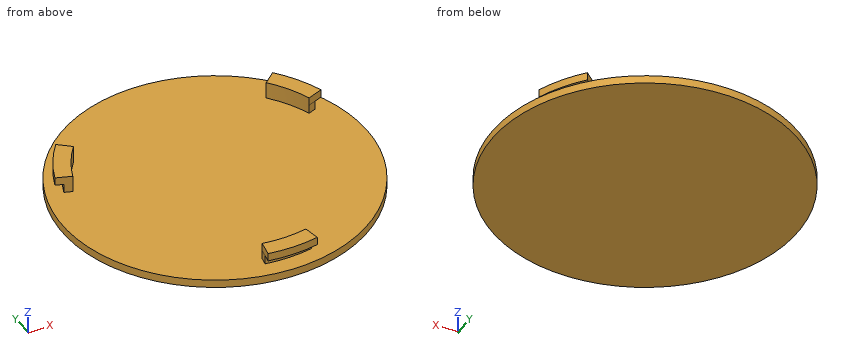
from build123d import *

# Parameters (mm, degrees)
F0_R     = 19
F1_DEPTH = 1
F3_DEPTH = 1.1
F5_DEPTH = 1


with BuildPart() as f1:
    # F0 (on Top) → F1 (new body)
    with BuildSketch(Plane.XY):
        Circle(F0_R)
    extrude(amount=F1_DEPTH)

    # F2 (on face) → F3 (join)
    with BuildSketch(Plane.XY.offset(1)):
        with BuildLine():
            Line((14.815816, 5.770752), (15.747629, 6.133693))
            ThreePointArc((15.747629, 6.133693), (14.443282, 8.775055), (12.700084, 11.149792))
            Line((12.700084, 11.149792), (11.9486, 10.490041))
            ThreePointArc((11.9486, 10.490041), (13.58865, 8.255821), (14.815816, 5.770752))
        make_face()
        with BuildLine():
            ThreePointArc((-15.058942, 5.102771), (-13.944076, 7.640206), (-12.405526, 9.945497))
            Line((-12.405526, 9.945497), (-13.185748, 10.571))
            ThreePointArc((-13.185748, 10.571), (-14.821062, 8.120722), (-16.006045, 5.4237))
            Line((-16.006045, 5.4237), (-15.058942, 5.102771))
        make_face()
        with BuildLine():
            ThreePointArc((3.110342, -15.592812), (0.355426, -15.896027), (-2.41029, -15.71625))
            Line((-2.41029, -15.71625), (-2.561881, -16.704693))
            ThreePointArc((-2.561881, -16.704693), (0.377779, -16.895777), (3.305961, -16.573492))
            Line((3.305961, -16.573492), (3.110342, -15.592812))
        make_face()
    extrude(amount=F3_DEPTH)

    # F4 (on face) → F5 (join)
    with BuildSketch(Plane.XY.offset(2.1)):
        with BuildLine():
            ThreePointArc((-15.058942, 5.102771), (-13.944076, 7.640206), (-12.405526, 9.945497))
            Line((-12.405526, 9.945497), (-13.96597, 11.196503))
            ThreePointArc((-13.96597, 11.196503), (-15.698048, 8.601238), (-16.953148, 5.744629))
            Line((-16.953148, 5.744629), (-15.058942, 5.102771))
        make_face()
        with BuildLine():
            Line((-2.41029, -15.71625), (-2.713471, -17.693136))
            ThreePointArc((-2.713471, -17.693136), (0.400133, -17.895527), (3.50158, -17.554172))
            Line((3.50158, -17.554172), (3.110342, -15.592812))
            ThreePointArc((3.110342, -15.592812), (0.355426, -15.896027), (-2.41029, -15.71625))
        make_face()
        with BuildLine():
            Line((14.815816, 5.770752), (16.679441, 6.496633))
            ThreePointArc((16.679441, 6.496633), (15.297915, 9.294289), (13.451568, 11.809543))
            Line((13.451568, 11.809543), (11.9486, 10.490041))
            ThreePointArc((11.9486, 10.490041), (13.58865, 8.255821), (14.815816, 5.770752))
        make_face()
    extrude(amount=F5_DEPTH)


solid = f1.part
Model file for the job. Use its own axes, mm. Round coordinates to 2 decimals unless told otherwise and drop trailing zeros. Loops run counter-clockwise (first coordinate to the right, second up) from the corner with the lowest first, then second, coordinate; pieces in that order, holes last. Notation, with made-up numbers: (36.5, 81.25) - (83.5, 81.25) arc R21 ccw to (83.5, 116.25) - close; hole circle Ø1 at (87, -11.75). An arc over 180 degrees is marked (long way). Write each question's results on one line, items separated by ' | '.
(1) Saw through at B-B, the plane y = 0. List the corners of the cut face in (x, z), then the cut area to 3 significant figures.
Answer below:
outline: (-19, 0) - (19, 0) - (19, 1) - (-19, 1) - close | area: 38.0 mm^2
(2) Pin check, flat tips, straight feed: pin 1 (11.5 mm diameter, centred on x = 3.5, y = 8, fed in from +Z); pin 2 (1.5 mm diameter, centred on y = 4, z = 0.5, fed in from -X). Stop position of each tip, or through.
Answer below:
pin 1: stops at z = 1 | pin 2: stops at x = -18.72
(3) Saw through at A-A, the plane x = 0. List the corners of the cut face in (y, z).
Answer below:
outline: (-19, 0) - (19, 0) - (19, 1) - (-15.9, 1) - (-15.9, 3.1) - (-17.9, 3.1) - (-17.9, 2.1) - (-16.9, 2.1) - (-16.9, 1) - (-19, 1) - close
(4) Wall check: L1, parallel to Z at x = -9, y = 1.5; L2, parallel to X at y = 12.5, z = 0.7; L3, parallel to Y at x = -1, z = 1.1. Give the ranges that are in metal, low to high.
Answer below:
L1: z = 0 to 1 | L2: x = -14.31 to 14.31 | L3: y = -16.87 to -15.87
(5) Saw through at C-C, the plane x = -7.5. List the corners of the cut face in (y, z), then the cut area to 3 significant figures.
Answer below:
outline: (-17.46, 0) - (17.46, 0) - (17.46, 1) - (-17.46, 1) - close | area: 34.9 mm^2
